Check sheet for the drawn part. Datum: minimum x, y, z corner. Units: mm. Round coordinates to 2 decimals unless told otherwise and drop trailing zeros. Write each loop counter-clockwise with the first axis right and the second up, starting at its lowest first coordinate (ties: lowest second). Pieces come first, ordered by that corner, then holes.
Item 1: Cross-section at C-C on x = 65.95. Enter the section's corners in (y, z).
Item 2: Cross-section at A-A on z = 0.45. Enter the section's corners in (x, y).
Item 3: Material ranges on line 1 (Y direction, x = 69, z = 1.3); line 2 (Y direction, x = 7.05, z = 1.6); line 3 (X direction, y = 47, z = 0.45), recorded low to high.
Item 4: Cross-section at B-B on x = 4. Enter the section's corners in (y, z).
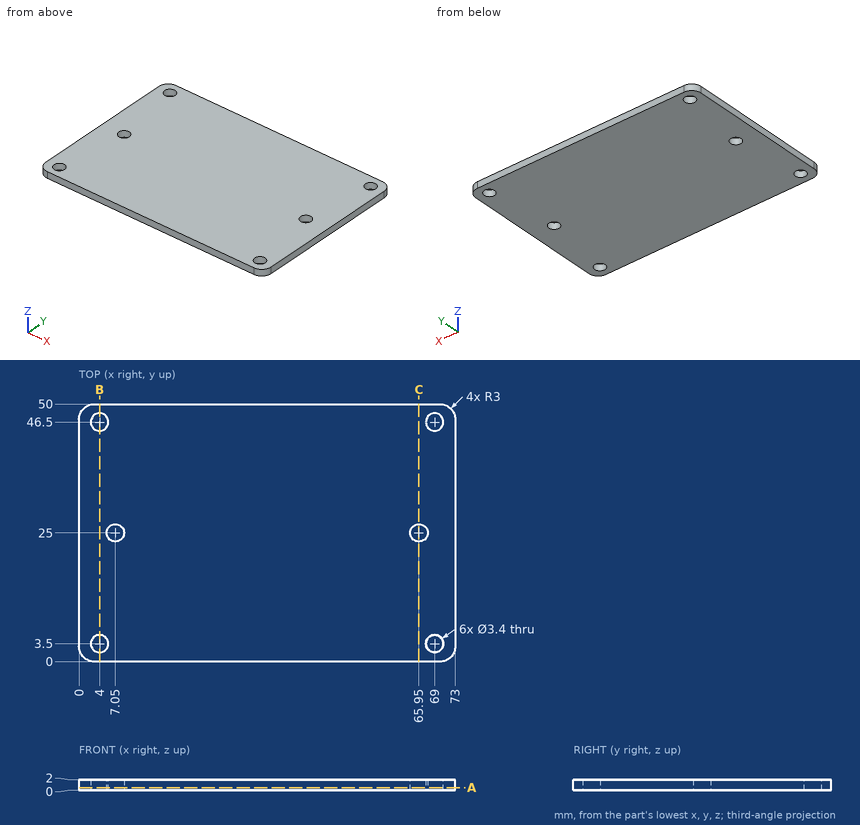
Response values:
1. outline: (0, 0) - (23.3, 0) - (23.3, 2) - (0, 2) - close; (26.7, 0) - (50, 0) - (50, 2) - (26.7, 2) - close
2. outline: (0, 3) arc R3 ccw to (3, 0) - (70, 0) arc R3 ccw to (73, 3) - (73, 47) arc R3 ccw to (70, 50) - (3, 50) arc R3 ccw to (0, 47) - close; hole circle Ø3.4 at (4, 3.5); hole circle Ø3.4 at (4, 46.5); hole circle Ø3.4 at (7.05, 25); hole circle Ø3.4 at (65.95, 25); hole circle Ø3.4 at (69, 3.5); hole circle Ø3.4 at (69, 46.5)
3. line 1: y = 0 to 1.8, 5.2 to 44.8, 48.2 to 50
3. line 2: y = 0 to 23.3, 26.7 to 50
3. line 3: x = 0 to 2.38, 5.62 to 67.38, 70.62 to 73
4. outline: (0, 0) - (1.8, 0) - (1.8, 2) - (0, 2) - close; (5.2, 0) - (44.8, 0) - (44.8, 2) - (5.2, 2) - close; (48.2, 0) - (50, 0) - (50, 2) - (48.2, 2) - close
